Autodesk Inventor part; units mm, degrees
ref_plane "YZ Plane" through (0, 0, 0) normal (1, 0, 0) x (0, 1, 0)
ref_plane "XZ Plane" through (0, 0, 0) normal (0, 1, 0) x (-1, 0, 0)
ref_plane "XY Plane" through (0, 0, 0) normal (0, 0, 1) x (1, 0, 0)
sketch "Sketch1" plane through (0, 0, 0) normal (0, 0, 1) x (1, 0, 0)
  arc A0 (10, 0) -> (0, 0) centre (5, -3.3166) ccw
  arc A1 (0, 203.3668) -> (10, 203.3668) centre (5, 206.6834) ccw
  line L0 (0, 203.3668) -> (0, 0)
  line L1 (10, 0) -> (10, 203.3668)
  dimension "d0" = 10
  dimension "d1" = 6
  dimension "d2" = 210
extrude "Extrusion1" add sketch "Sketch1" along normal blind 3.175
sketch "Sketch2" plane through (0, 0, 3.175) normal (0, 0, 1) x (1, 0, 0)
  arc A0 (10, 0) -> (0, 0) centre (5, -3.3166) ccw
  arc A1 (0, 203.3668) -> (10, 203.3668) centre (5, 206.6834) ccw
  line L0 (0, 203.3668) -> (0, 0)
  line L1 (2.4125, 2.0968) -> (2.4125, 2.6834)
  line L2 (2.4125, 2.6834) -> (3.4125, 2.6834)
  line L3 (3.4125, 2.6834) -> (3.4125, 100.0959)
  line L4 (3.4125, 101.6834) -> (6.5875, 101.6834)
  line L5 (6.5875, 100.0959) -> (6.5875, 2.6834)
  line L6 (6.5875, 2.6834) -> (7.5875, 2.6834)
  line L7 (7.5875, 2.6834) -> (7.5875, 2.0968)
  arc A2 (3.4125, 101.6834) -> (3.4125, 100.0959) centre (3.4125, 100.8896) ccw
  arc A3 (6.5875, 100.0959) -> (6.5875, 101.6834) centre (6.5875, 100.8896) ccw
  line L8 (10, 0) -> (10, 203.3668)
  line L9 (2.4125, 201.27) -> (2.4125, 200.6834)
  line L10 (2.4125, 200.6834) -> (7.5875, 200.6834)
  line L11 (7.5875, 200.6834) -> (7.5875, 201.27)
  point P0 (5, 101.6834)
  dimension "d6" = 3.175
  dimension "d7" = 1
  dimension "d8" = 210
  dimension "d9" = 105
  dimension "d10" = 0.7937
extrude "Extrusion2" cut sketch "Sketch2" against normal up to next contours A0 L1 L2 L3 A2 L4 A3 L5 L6 L7 | L11 L10 A1 | L10 L9 A1
fillet "Fillet1" radius 0.7937 4 edges at (2.4125, 2.6834, 1.5875) (7.5875, 2.6834, 1.5875) (2.4125, 200.6834, 1.5875) (7.5875, 200.6834, 1.5875)
fillet "Fillet1" radius 0.5 4 edges at (0, 0, 1.5875) (10, 0, 1.5875) (10, 203.3668, 1.5875) (0, 203.3668, 1.5875)
equation "\"d3\" = THICKA"
equation "\"d6\" = THICKA"
equation "\"d9\" = 0.5 * d8"
equation "\"d11\" = THICKA"
equation "\"THICKA\" = 3.175"
equation "\"THICKB\" = 6.731"
equation "\"THICKC\" = 12.7"
equation "\"MAGDIA\" = 9.5"
equation "\"BALLDIA\" = 12"
properties part number "Effector_Arm_Ball"
Build history of the part. All positions in model axes, mm. A direction names the side the tool comes from. Round coordinates to 2 decimals unless told otherwise and drop trailing zeros. Write each loop counter-clockwise with the first axis right and the second up, starting at its lowest first coordinate (ties: lowest second). Pieces come first, ordered by that corner, then holes. Notation, with made-up numbers: (-2.75, 32) -> (53.25, 32) arc R21 ccw to (53.25, 41) -> close; hole circle Ø11 at (56.25, 36.5). An arc over 180 degrees is marked (long way). Write item = value, one per line.
(1) Band-saw the part on B-B (z = 0.55). Give the cut face in (x, y), then the cut area to 3 significant figures.
Answer:
outline = (0, 1.37) arc R0.5 ccw to (0.85, 1.01) arc R6 cw to (2.41, 2.1) arc R0.79 cw to (3.18, 2.68) -> (3.41, 2.68) -> (3.41, 100.1) arc R0.79 cw to (3.41, 101.68) -> (6.59, 101.68) arc R0.79 cw to (6.59, 100.1) -> (6.59, 2.68) -> (6.82, 2.68) arc R0.79 cw to (7.59, 2.1) arc R6 cw to (9.15, 1.01) arc R0.5 ccw to (10, 1.37) -> (10, 201.99) arc R0.5 ccw to (9.15, 202.35) arc R6 cw to (7.59, 201.27) arc R0.79 cw to (6.82, 200.68) -> (3.18, 200.68) arc R0.79 cw to (2.41, 201.27) arc R6 cw to (0.85, 202.35) arc R0.5 ccw to (0, 201.99) -> close
area = 1,680 mm2
(2) Two-plate mould, pull along X, no slides. Class faces 4 (the face through (0, 103, 2)), 5 (the face through (5, 101.683, 2)), 6 (the face through (5, 103, 3.175)): pulls with the +X half, pulls with the -X half, needs draft (parallel to the pull), parting line crosses it, or undercut.
Answer:
face_4 = pulls with the -X half
face_5 = undercut
face_6 = needs draft
(3) Flat gauge pins, fed straight in: pin 1 (1.6 mm diameter, centred on x = 5, z = 1, fed in from -Y); pin 2 (1.6 mm diameter, centred on x = 5.5, z = 1, fed in from +Y). Where does each tip first touch, or does it go through?
Answer:
pin_1 = 101.68
pin_2 = 200.68
(4) Band-saw the part on A-A (y = 43.5). Give the cut face in (x, z) (1 decimal).
Answer:
outline = (0, 0) -> (3.4, 0) -> (3.4, 3.2) -> (0, 3.2) -> close; (6.6, 0) -> (10, 0) -> (10, 3.2) -> (6.6, 3.2) -> close
(5) Probe L1, parallel to X at y = 86, z = 0.3; L2, parallel to Y at x = 3, z = 1.25; L3, parallel to Y at x = 2.75, z = 0.8. List the from-to ranges inside material, lowest first.
Answer:
L1 = 0 to 3.41, 6.59 to 10
L2 = 2.66 to 100.21, 101.57 to 200.7
L3 = 2.56 to 100.45, 101.33 to 200.81
(6) Tool access for faces 1 (the face through (6.588, 52, 2)), 2 (the face through (5, 200.683, 2)), 3 (the face through (10, 100, 2)): list every direction of +Z, -Z, +X, -X, +Y, -Y with a clear straight run to the whole face (end or side of a thin tool).
Answer:
face_1 = +Z, -Z, -Y
face_2 = +Z, -Z, +Y
face_3 = +Z, -Z, +X, +Y, -Y
